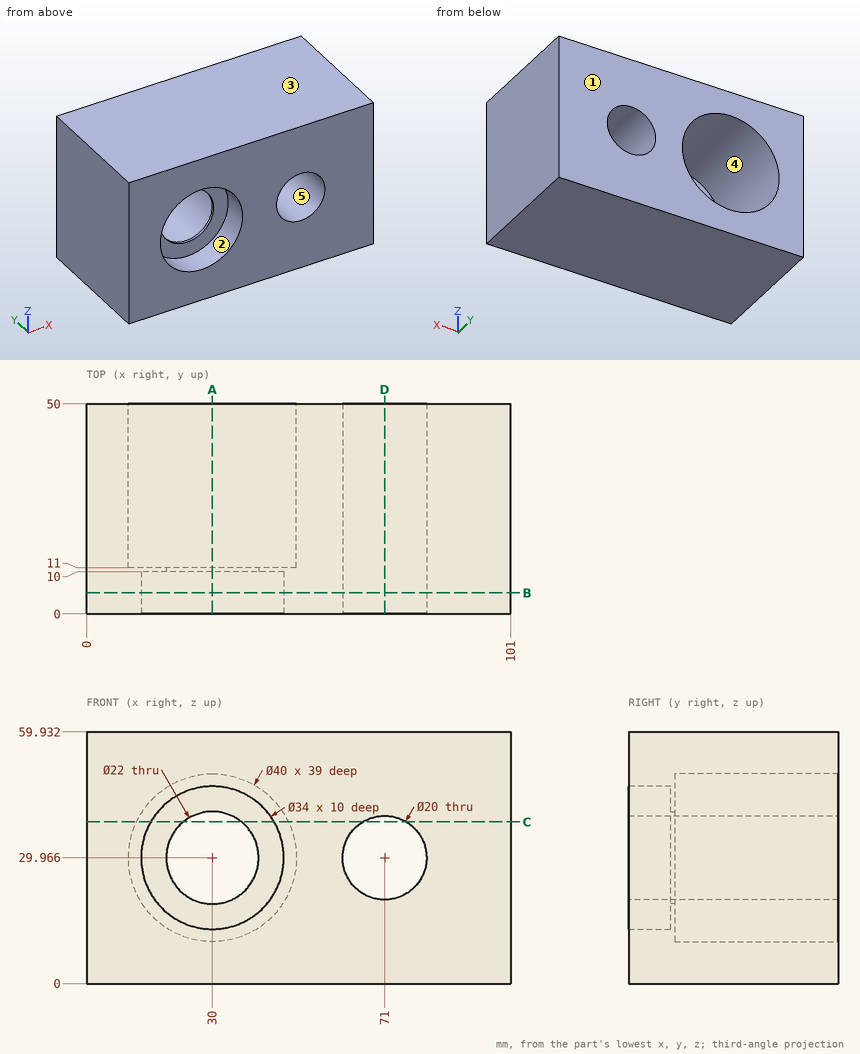
Part print with two shaded views. Sizes in mm from the minimum x, y, z corner. A direction names the side the tool comes from. Coordinates: 2 decimals unless noted, no trailing zeros. Order: outer loops, then holes, each group sorted by start corner. A loop starts at its lowest first (then second) coordinate and runs counter-clockwise, first axis right, second up. Notation, with made-up numbers: M 55,70.5 L 101,70.5 A13 cw 101,91.5 Z; hole C -21.5,28.5 d7. An arc over 180 degrees is marked long. Use a Markdown table: item, result.
(1) Probe L1, parallel to Z at x = 30, y = 10.35; L2, parallel to X at y = 43, z = 23.5; L3, parallel to Z at x = 75, y = 35.5. List the from-to ranges inside material, lowest first.
A:
| item | result |
|---|---|
| L1 | z = 0 to 18.97, 40.97 to 59.93 |
| L2 | x = 0 to 11.07, 48.93 to 63.37, 78.63 to 101 |
| L3 | z = 0 to 20.8, 39.13 to 59.93 |
(2) Pull direction Z, two halves, no side cores. Call the marked faces 1, 2 and 3: released by +Z, released by -Z, zero draft, split by the parting line, or undercut.
A:
| item | result |
|---|---|
| face 1 | zero draft |
| face 2 | undercut |
| face 3 | released by +Z |
(3) Tool access for the marked faces 4 and 5: list every direction of +Z, -Z, +X, -X, +Y, -Y with a clear straight run to the whole face (end or side of a thin tool).
A:
| item | result |
|---|---|
| face 4 | +Y |
| face 5 | +Y, -Y |
(4) Cut at A-A on x = 30. Write the cut outline in (y, z), then the cut area to 3 significant figures.
A:
| item | result |
|---|---|
| outline | M 0,0 L 50,0 L 50,9.97 L 11,9.97 L 11,18.97 L 10,18.97 L 10,12.97 L 0,12.97 Z; M 0,46.97 L 10,46.97 L 10,40.97 L 11,40.97 L 11,49.97 L 50,49.97 L 50,59.93 L 0,59.93 Z |
| area | 1,070 mm^2 |
(5) Cut at D-D on x = 71. Write the cut outline in (y, z).
A:
| item | result |
|---|---|
| outline | M 0,0 L 50,0 L 50,19.97 L 0,19.97 Z; M 0,39.97 L 50,39.97 L 50,59.93 L 0,59.93 Z |
(6) Cut at B-B on y = 5. Write the cut outline in (x, z), then the cut area to 3 significant figures.
A:
| item | result |
|---|---|
| outline | M 0,0 L 101,0 L 101,59.93 L 0,59.93 Z; hole C 30,29.97 d34; hole C 71,29.97 d20 |
| area | 4,830 mm^2 |
(7) Flat gauge pin, fed straight in: pin 1 (24 mm diameter, centred on x = 30, z = 29.97, fed in from -Y). Where does the tip first touch, or does it go through?
A:
| item | result |
|---|---|
| pin 1 | stops at y = 10 |
(8) Cut at C-C on z = 38.5. Write the cut outline in (x, y).
A:
| item | result |
|---|---|
| outline | M 0,0 L 15.3,0 L 15.3,10 L 23.06,10 L 23.06,11 L 11.91,11 L 11.91,50 L 0,50 Z; M 36.94,10 L 44.7,10 L 44.7,0 L 65.79,0 L 65.79,50 L 48.09,50 L 48.09,11 L 36.94,11 Z; M 76.21,0 L 101,0 L 101,50 L 76.21,50 Z |
